```python
from build123d import *

# Parameters (mm, degrees)
F0_R     = 2.335
F1_DEPTH = 33.02
F2_R     = 5.08
F2_R_2   = 2.335
F3_DEPTH = 2.54
F4_R     = 0.889
F5_DEPTH = 12.7


with BuildPart() as f1:
    # F0 (on Top) → F1 (new body)
    with BuildSketch(Plane.XY):
        Circle(F0_R)
    extrude(amount=F1_DEPTH)

    # F2 (on face) → F3 (join)
    with BuildSketch(Plane(origin=(0, 0, 0), x_dir=(1, 0, 0), z_dir=(0, 0, -1))):
        Circle(F2_R)
        Circle(F2_R_2, mode=Mode.SUBTRACT)
        Circle(F2_R_2)
    extrude(amount=F3_DEPTH)

    # F4 (on Front) → F5 (cut, symmetric)
    with BuildSketch(Plane.XZ):
        with Locations((0, 31.369)):
            Circle(F4_R)
    extrude(amount=F5_DEPTH, both=True, mode=Mode.SUBTRACT)


solid = f1.part
```
CAD build for the part. Positions are in the model's coordinates, mm. A direction names the side the tool comes from. Give positions to 0.01 mm unless a question says otherwise; leave off trailing zeros. Order: outer loops, then holes, each group sorted by start corner. A loop starts at its lowest first (then second) coordinate and runs counter-clockwise, first axis right, second up.
(1) Saw through at A-A, the plane x = 0. Give the cut face in (y, z) (3 decimals).
(2) Drill centre lines: L1, parallel to Z at x = 0, y = -1.1; L2, parallel to Z at x = -1, y = 3.5; L3, parallel to Y at x = 0, z = 22 (3 decimals). Where is each one in solid material? Low to high.
(3) Saw through at D-D, the plane y = 3.25. Give the cut face in (x, z), then the cut area to 3 significant figures.
(4) Mould opens along Z. For faces 3 (the flat face through (0, 0, -2.54)), 4 (the cylindrical face through (-0.19, -0.03, 30.5)), 5 (the flat face through (2.2, -1.2, 0)) say: released by +Z, released by -Z, zero draft, split by the parting line, or undercut.
(5) Flat gauge pins, fed straight in: pin 1 (4 mm diameter, centred on x = -3, z = 9.5, fed in from +Y); pin 2 (3 mm diameter, centred on x = 1.5, z = 8, fed in from -Y) (3 decimals). Where does each tip first touch, or does it go through?
(6) Saw through at C-C, the plane z = 21.5. Give the cut face in (x, y) (3 decimals).
(7) Saw through at B-B, the plane y = -0.5. Give the cut face in (x, z), then the cut area to 3 significant figures.
(8) Tool access for faces 1 (the flat face through (0, 0, 33.02)), 2 (the cylindrical face through (2.16, -0.89, 16.28)): list every direction of +Z, -Z, +X, -X, +Y, -Y with a clear straight run to the whole face (end or side of a thin tool).
Results found:
1. outline: (-5.08, -2.54) - (5.08, -2.54) - (5.08, 0) - (2.335, 0) - (2.335, 30.48) - (-2.335, 30.48) - (-2.335, 0) - (-5.08, 0) - close; (-2.335, 32.258) - (2.335, 32.258) - (2.335, 33.02) - (-2.335, 33.02) - close
2. L1: z = -2.54 to 30.48, 32.26 to 33.02
2. L2: z = -2.54 to 0
2. L3: y = -2.335 to 2.335
3. outline: (-3.9, -2.54) - (3.9, -2.54) - (3.9, 0) - (-3.9, 0) - close
3. area: 19.8 mm2
4. face 3: released by -Z
4. face 4: undercut
4. face 5: released by +Z
5. pin 1: stops at y = 2.11
5. pin 2: stops at y = -2.335
6. outline: circle Ø4.67 at (0, 0)
7. outline: (-5.06, -2.54) - (5.06, -2.54) - (5.06, 0) - (2.28, 0) - (2.28, 33.02) - (-2.28, 33.02) - (-2.28, 0) - (-5.06, 0) - close; hole circle Ø1.78 at (0, 31.37)
7. area: 174 mm2
8. face 1: +Z, +X, -X, +Y, -Y
8. face 2: +Z
